Answer from the drawing. Dimensions are ordinates in mm from the lowest x, y and z of the part. A direction names the side the tool comes from. Coordinates: 2 decimals unless noted, no trailing zeros. Loops run counter-clockwise (first coordinate to the right, second up) from the corner with the lowest first, then second, coordinate; pieces in that order, holes last. Notation, with made-up numbers: (-7.5, 10.25) - (20.5, 10.25) arc R19 cw to (20.5, 36.25) - close; hole circle Ø1 at (45.5, 63). An arc over 180 degrees is marked (long way). Write each question's results on one line, items separated by ' | '. Start each with the question number.
1. Each of these flat-tipped pins is pushed along its axis until it touches: P1, Ø1.5, axis at x = 152.5, y = 124.5, coming from the +Z side; P2, Ø4, axis at y = 114.5, z = 40.5, coming from the +X side. Where does it stop, or does it pass through?
2. A cutting plane is placed at C-C on y = 82. Determine the outline of the cut face in (x, z), then the cut area to 3 significant figures.
3. A cutting plane is placed at B-B on z = 49. Determine the outline of the cut face in (x, y).
4. Which of the six approach directions +Z, -Z, +X, -X, +Y, -Y give full straight-line access (tool end or side, diameter ignored) to the marked faces 1, 2, 3 and 4?
5. A cutting plane is placed at A-A on x = 119. Determine the outline of the cut face in (y, z).
6. A cutting plane is placed at D-D on z = 13. Determine the outline of the cut face in (x, y), then the cut area to 3 significant figures.
7. Find the intervals of material crossed by line 1 along Z through (x, y) = (48.5, 89); line 2 along X through (y, z) = (110, 31.5); line 3 along Z through (x, y) = (113, 153.5), in increasing order. Write a range as [from, to].
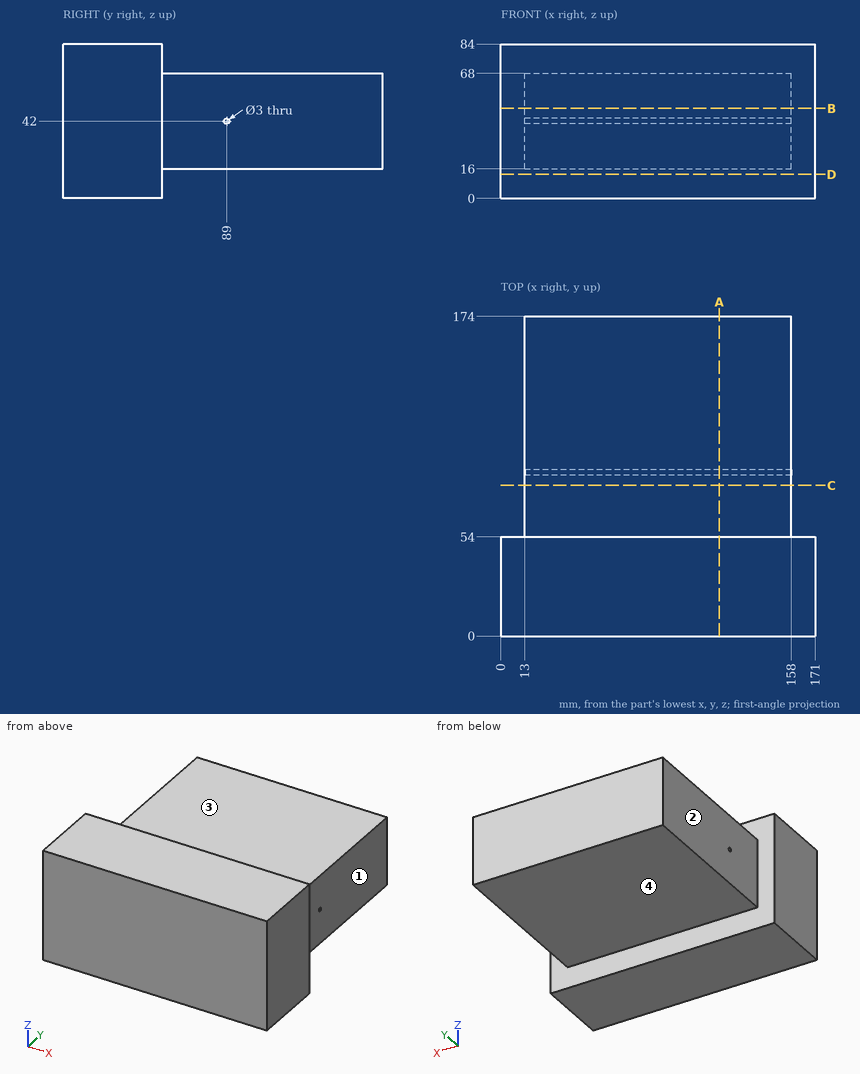
Values:
1) P1: z = 68 | P2: x = 158
2) outline: (13, 16) - (158, 16) - (158, 68) - (13, 68) - close | area: 7,540 mm^2
3) outline: (0, 0) - (171, 0) - (171, 54) - (158, 54) - (158, 174) - (13, 174) - (13, 54) - (0, 54) - close
4) face 1: +Z, -Z, +X, +Y | face 2: +Z, -Z, -X, +Y | face 3: +Z, +X, -X, +Y | face 4: -Z, +X, -X, +Y
5) outline: (0, 0) - (54, 0) - (54, 16) - (174, 16) - (174, 68) - (54, 68) - (54, 84) - (0, 84) - close; hole circle Ø3 at (89, 42)
6) outline: (0, 0) - (171, 0) - (171, 54) - (0, 54) - close | area: 9,230 mm^2
7) line 1: [16, 40.5], [43.5, 68] | line 2: [13, 158] | line 3: [16, 68]
